Verification items for the finished model (mm, model axes). Face numbers are marked on the shaded views. A direction names the side the tool comes from. Give positions to 0.01 mm unless a question says otherwise; leave off trailing zeros. Order: outer loops, then holes, each group sorted by start corner. A loop starts at its lowest first (then second) coordinate and runs counter-clockwise, first axis right, second up. Notation, with made-up numbers: (17.25, 76) -> (39.25, 76) arc R21 ccw to (39.25, 114) -> close; hole circle Ø6 at (44, 54.5). An arc over 180 degrees is marked (long way). Return JSON: item names as keys, results as strings. Group by question number.
(1) Cross-section at A-A on z = 0. Enter the section's corners in (x, y), then the cut area to 3 significant figures.
(2) Cross-section at B-B on x = -0.2. Enter the section's corners in (y, z), then the cut area to 3 significant figures.
(3) Tool access check on the marked faces 1, 2 and 3. Record the directions out of +Z, -Z, +X, -X, +Y, -Y that give a thin tool (end or side, any length) a straight path to the whole face; none if there is none.
(4) Depth check by flat-ended pin: pin 1 Ø1.5 at (y, z) = (20, 2) entering from -X. Enter the tip coordinate at first touch or a pass-through.
(5) Cross-section at C-C on y = 22.25. Enter the section's corners in (x, z), then the cut area to 3 significant figures.
(6) Cross-section at D-D on y = 3.5. Enter the section's corners in (x, z).
(7) Thickness scan on line 1 along Y through (x, z) = (1, 1.7); line 2 along Y through (x, z) = (0.9, -1.25); line 3 along Z through (x, y) = (-1, 16.5). Record the ranges inside material, lowest first.
from build123d import *

# Parameters (mm, degrees)
SKETCH_2_W   = 1.5
SKETCH_2_H   = 10
SKETCH_2_W_2 = 1.489718874


with BuildPart() as part:
    # 草图2 → 旋转1 (revolve)
    with BuildSketch(Plane(origin=(0, 0, 0), x_dir=(0, 0, -1), z_dir=(1, 0, 0))):
        with Locations((0.75, 5)):
            Rectangle(SKETCH_2_W, SKETCH_2_H)
        Polygon((0, 11.333239566), (0, 10), (1.5, 10), (1.852020266, 10), (1.852020266, 11.333239566), align=None)
        Polygon((0, 12.799080051), (0, 11.333239566), (1.852020266, 11.333239566), (2.456922178, 11.333239566), (2.456922178, 12.799080051), (1.898093602, 12.799080051), align=None)
        Polygon((0, 14.00271083), (0, 12.799080051), (1.898093602, 12.799080051), (1.898093602, 14.00271083), (1.489718874, 14.00271083), align=None)
        with Locations((0.744859437, 19.00271083)):
            Rectangle(SKETCH_2_W_2, SKETCH_2_H)
    revolve(axis=Axis((0, 0, 0), (0, 1, 0)))


solid = part.part
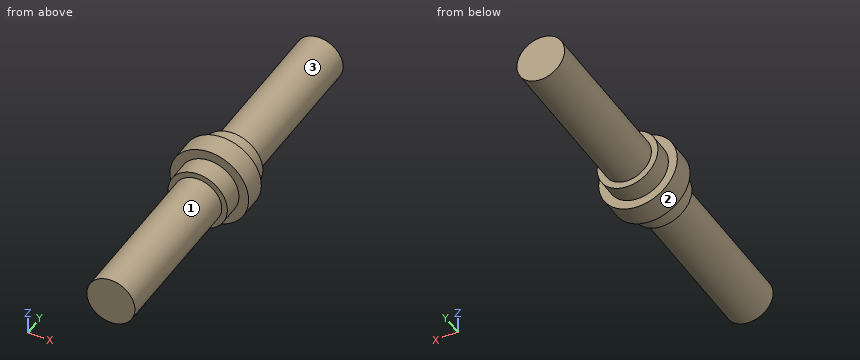
Verdict:
{
 "1": {"outline": "(-2.46, 11.33) -> (-1.85, 11.33) -> (-1.85, 10) -> (-1.5, 10) -> (-1.5, 0) -> (1.5, 0) -> (1.5, 10) -> (1.85, 10) -> (1.85, 11.33) -> (2.46, 11.33) -> (2.46, 12.8) -> (1.9, 12.8) -> (1.9, 14) -> (1.49, 14) -> (1.49, 24) -> (-1.49, 24) -> (-1.49, 14) -> (-1.9, 14) -> (-1.9, 12.8) -> (-2.46, 12.8) -> close", "area": "76.5 mm²"},
 "2": {"outline": "(0, -1.49) -> (10, -1.49) -> (10, -1.84) -> (11.33, -1.84) -> (11.33, -2.45) -> (12.8, -2.45) -> (12.8, -1.89) -> (14, -1.89) -> (14, -1.48) -> (24, -1.48) -> (24, 1.48) -> (14, 1.48) -> (14, 1.89) -> (12.8, 1.89) -> (12.8, 2.45) -> (11.33, 2.45) -> (11.33, 1.84) -> (10, 1.84) -> (10, 1.49) -> (0, 1.49) -> close", "area": "75.9 mm²"},
 "3": {"face 1": "-Y", "face 2": "+Y, -Y", "face 3": "+Y"},
 "4": {"pin 1": "x = -0.81"},
 "5": {"outline": "circle Ø2.98 at (0, 0)", "area": "6.97 mm²"},
 "6": {"outline": "circle Ø3 at (0, 0)"},
 "7": {"line 1": "11.33 to 12.8", "line 2": "10 to 14", "line 3": "-1.1 to 1.1"}
}
